Source: CAD feature listing. Evaluate the final solid. Frame: model axes, mm. Face numbers are marked on the shaded views. A direction names the side the tool comes from. Round coordinates to 2 decimals unless told otherwise and drop trailing zeros. Order: outer loops, then holes, each group sorted by start corner. A loop starts at its lowest first (then second) coordinate and runs counter-clockwise, first axis right, second up. Notation, with made-up numbers: M 36.25,50.5 L 52.25,50.5 A18 cw 52.25,64.5 Z; hole C -26,71.25 d5. An arc over 180 degrees is marked long. Use one line per item in the form item = value. Start each with the question number.
Q1. Contact query for flat-ended pins moving along their axis: pin 1 (6.5 mm diameter, centred on x = 0, y = 10, fed in from +Z); pin 2 (3 mm diameter, centred on x = 0, y = -10, fed in from -Z); pin 3 (8 mm diameter, centred on y = 5.5, z = 8.5, fed in from -X); pin 4 (5 mm diameter, centred on y = -1, z = 12.5, fed in from +X). Output: stop coordinate, or through.
Q2. Section A-A (x = 0). Return the cut outline in (y, z), plus the area to 3 significant figures.
Q3. Section C-C (x = 8.5). Return the cut outline in (y, z), plus the area to 3 significant figures.
Q4. Material intervals for probe 1 along Y at (x, z) = (0, 0.7); probe 2 along Z at (x, y) = (-3.75, 9); probe 3 along Y at (x, z) = (10, 1.15), sorted ascending.
Q5. Section D-D (y = -10). Return the cut outline in (x, z), plus the area to 3 significant figures.
Q6. Reachability of the marked faces 1 and 2 from +Z, -Z, +X, -X, +Y, -Y: full face, straight path, thin tool, end or side. Return the list, or none.
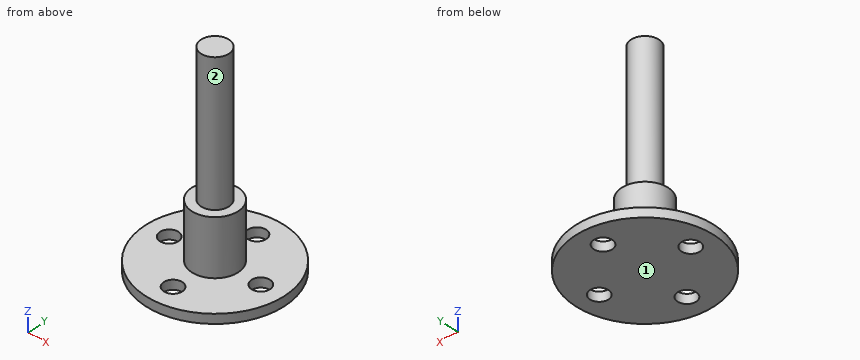
from build123d import *

# Parameters (mm, degrees)
SKETCH1_R           = 15
BOSS_EXTRUDE1_DEPTH = 2
SKETCH2_R           = 5
BOSS_EXTRUDE2_DEPTH = 12
SKETCH3_R           = 2
CUT_EXTRUDE1_DEPTH  = 6
SKETCH4_R           = 3
BOSS_EXTRUDE3_DEPTH = 30


with BuildPart() as part:
    # Sketch1 → Boss-Extrude1 (new body)
    with BuildSketch(Plane.XY):
        Circle(SKETCH1_R)
    extrude(amount=BOSS_EXTRUDE1_DEPTH)

    # Sketch2 → Boss-Extrude2 (add)
    with BuildSketch(Plane.XY.offset(2)):
        Circle(SKETCH2_R)
    extrude(amount=BOSS_EXTRUDE2_DEPTH)

    # Sketch3 → Cut-Extrude1 (cut)
    with BuildSketch(Plane.XY.offset(2)):
        with Locations((0, 10)):
            Circle(SKETCH3_R)
        with Locations((10, 0)):
            Circle(SKETCH3_R)
        with Locations((0, -10)):
            Circle(SKETCH3_R)
        with Locations((-10, 0)):
            Circle(SKETCH3_R)
    extrude(amount=-CUT_EXTRUDE1_DEPTH, mode=Mode.SUBTRACT)

    # Sketch4 → Boss-Extrude3 (add)
    with BuildSketch(Plane.XY.offset(14)):
        Circle(SKETCH4_R)
    extrude(amount=BOSS_EXTRUDE3_DEPTH)


solid = part.part
Results list:
q1.pin_1 = 2
q1.pin_2 = through
q1.pin_3 = -4.77
q1.pin_4 = 5
q2.outline = M -15,0 L -12,0 L -12,2 L -15,2 Z; M -8,0 L 8,0 L 8,2 L 5,2 L 5,14 L 3,14 L 3,44 L -3,44 L -3,14 L -5,14 L -5,2 L -8,2 Z; M 12,0 L 15,0 L 15,2 L 12,2 Z
q2.area = 344 mm2
q3.outline = M -12.36,0 L -1.32,0 L -1.32,2 L -12.36,2 Z; M 1.32,0 L 12.36,0 L 12.36,2 L 1.32,2 Z
q3.area = 44.1 mm2
q4.probe_1 = -15 to -12, -8 to 8, 12 to 15
q4.probe_2 = 0 to 2
q4.probe_3 = -11.18 to -2, 2 to 11.18
q5.outline = M -11.18,0 L -2,0 L -2,2 L -11.18,2 Z; M 2,0 L 11.18,0 L 11.18,2 L 2,2 Z
q5.area = 36.7 mm2
q6.face_1 = -Z, +X, -X, +Y, -Y
q6.face_2 = +Z
